The drawing under review shows one solid part. Ordinate dimensions are in mm from its lowest x, y, z. A direction names the side the tool comes from. Give positions to 0.01 mm unless a question says otherwise; leave off trailing zeros. Loops run counter-clockwise (first coordinate to the right, second up) from the corner with the lowest first, then second, coordinate; pieces in that order, holes last. Notation, with made-up numbers: (-8.5, 56.5) -> (16.5, 56.5) arc R9 ccw to (16.5, 61.5) -> close; hole circle Ø2 at (60.5, 25.5). An arc over 180 degrees is marked (long way). Answer in a Markdown table with one row per item. Add a question column.
(1) Draft analysis for pull direction Z (two halves, no side actions). For the marked faces 1, 2, 3 and 4, state which applies: +Z half, -Z half, draft (parallel to the pull), parting line (faces both ways), or undercut.
(2) Consider section C-C on y = 3.75. Write out the cut boundary in (x, z).
(3) For pin 1 (1.8 mm diameter, centred on x = 5, y = 5, fed in from -Z); pin 2 (2.5 mm diameter, centred on y = 2, z = 4, fed in from -X); pin 3 (2.5 mm diameter, centred on x = 14, z = 3, fed in from +Y); pin 4 (5 mm diameter, centred on y = 1.5, z = 8, fed in from +X), all flat-tipped, find the tip position at first contact; note any pin that passes through.
(4) For line 1 (Z direction, x = 15, y = 1.7); line 2 (Y direction, x = 5, z = 0.75); line 3 (Z direction, x = 6, y = 2.75), list the stretches that pass through material, from the lowest coordinate up.
(5) Consider section A-A on x = 5. Write out the cut boundary in (y, z), then the cut area to 3 significant figures.
(6) For the marked faces 5, 6 and 7, list the 3-axis set-ups (+Z, -Z, +X, -X, +Y, -Y) from which the entire face can be reached by the end or side of a thin tool; tool diameter is ignored.
(7) Consider section D-D on z = 1. Write out the cut boundary in (x, y), then the cut area to 3 significant figures.
(8) Consider section B-B on y = 1.5. Write out the cut boundary in (x, z).
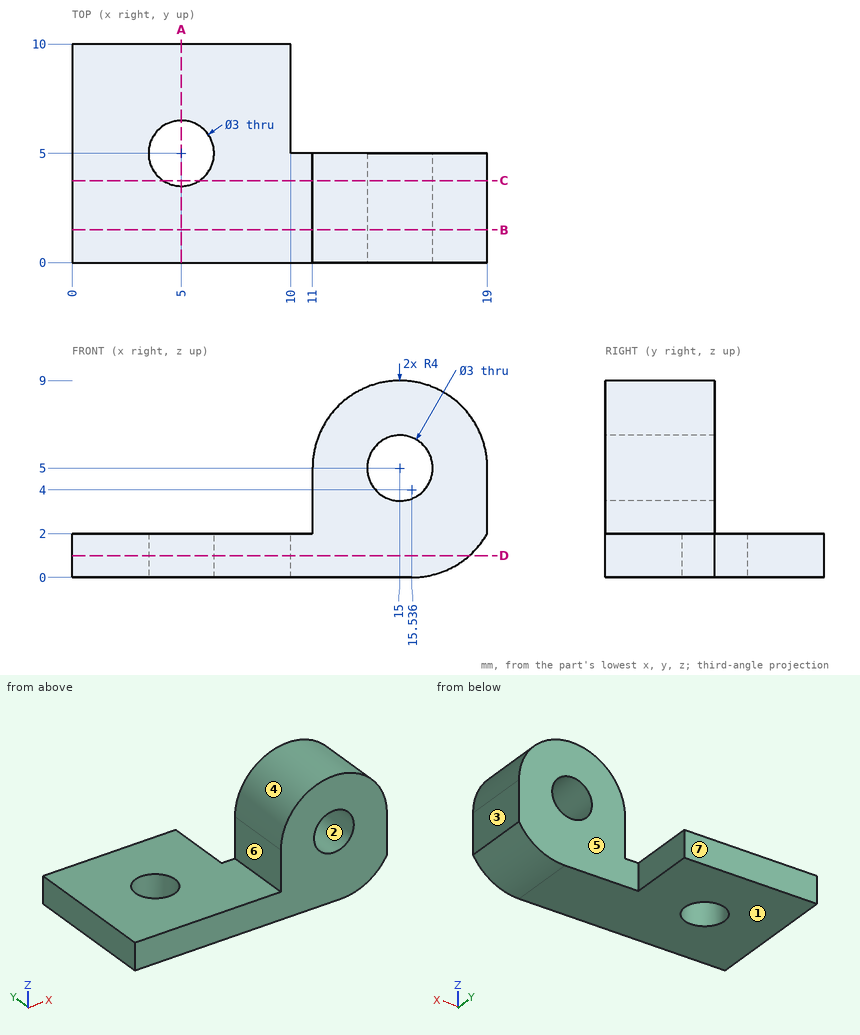
Values follow:
| question | item | result |
|---|---|---|
| 1 | face 1 | -Z half |
| 1 | face 2 | undercut |
| 1 | face 3 | draft |
| 1 | face 4 | +Z half |
| 2 | outline | (0, 0) -> (4.17, 0) -> (4.17, 2) -> (0, 2) -> close; (5.83, 0) -> (15.54, 0) arc R4 ccw to (19, 2) -> (19, 5) arc R4 ccw to (11, 5) -> (11, 2) -> (5.83, 2) -> close; hole circle Ø3 at (15, 5) |
| 3 | pin 1 | through |
| 3 | pin 2 | x = 11 |
| 3 | pin 3 | y = 5 |
| 3 | pin 4 | x = 18.97 |
| 4 | line 1 | 0 to 3.5, 6.5 to 9 |
| 4 | line 2 | 0 to 3.5, 6.5 to 10 |
| 4 | line 3 | 0 to 2 |
| 5 | outline | (0, 0) -> (3.5, 0) -> (3.5, 2) -> (0, 2) -> close; (6.5, 0) -> (10, 0) -> (10, 2) -> (6.5, 2) -> close |
| 5 | area | 14.0 mm2 |
| 6 | face 5 | +Z, -Z, +X, +Y |
| 6 | face 6 | +Z, -X, +Y, -Y |
| 6 | face 7 | +Z, -Z, +X, -X, +Y |
| 7 | outline | (0, 0) -> (18.18, 0) -> (18.18, 5) -> (10, 5) -> (10, 10) -> (0, 10) -> close; hole circle Ø3 at (5, 5) |
| 7 | area | 134 mm2 |
| 8 | outline | (0, 0) -> (15.54, 0) arc R4 ccw to (19, 2) -> (19, 5) arc R4 ccw to (11, 5) -> (11, 2) -> (0, 2) -> close; hole circle Ø3 at (15, 5) |
